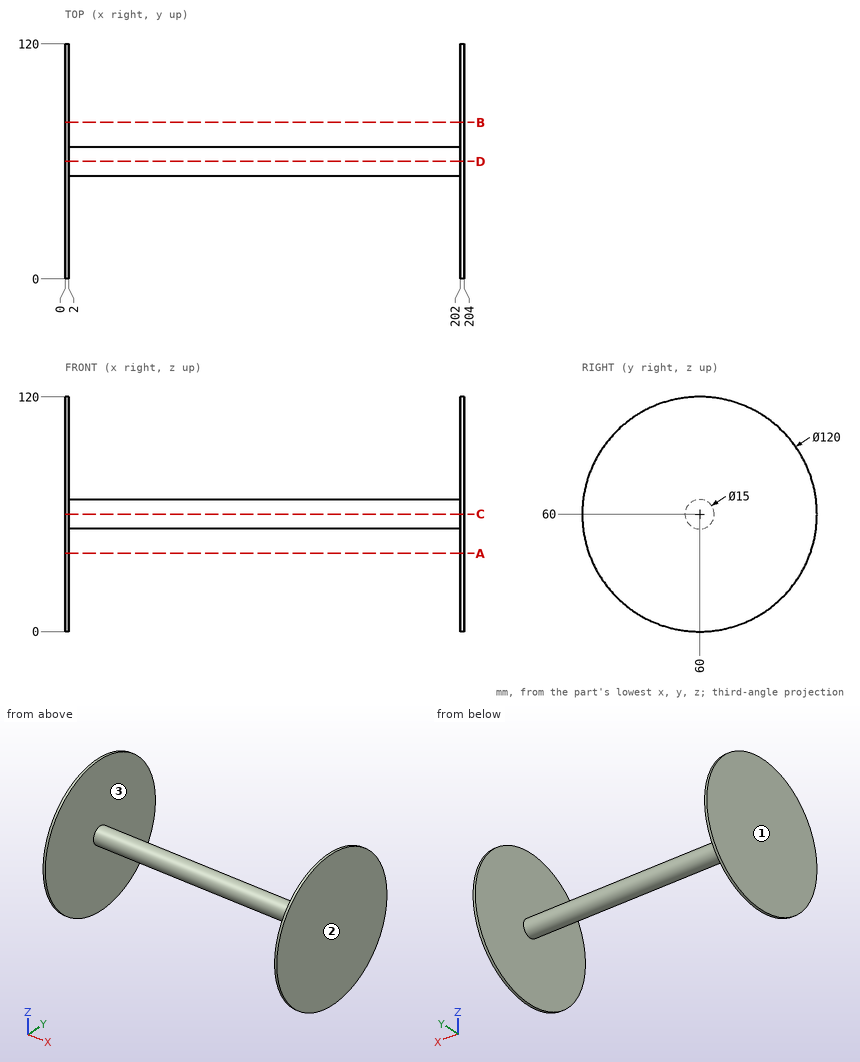
Design review of the part shown in the three views and the two pictorial views. Dimensions are in mm from the part's minimum x, y and z. Round coordinates to 2 decimals unless told otherwise and drop trailing zeros. Write each loop counter-clockwise with the first axis right and the second up, starting at its lowest first coordinate (ties: lowest second). Pieces come first, ordered by that corner, then holes. Notation, with made-up numbers: M -16,25 L 39,25 A19 cw 39,54 Z; hole C 53,5 d9. An arc over 180 degrees is marked long. Use a Markdown table: item, result. Add a question column.
Q1. To check wall thickness, follow line 1 (X direction, y = 92, z = 85). State the ranges of the line that lie inside material, in increasing order.
Q2. We need section C-C, the plane z = 60. State the section outline as (x, y) points, plus the area to 3 significant figures.
Q3. The part is to be moulded in two halves that separate along X. For the marked faces 1, 2 and 3, say which applies: pulls with the +X half, pulls with the -X half, needs draft (parallel to the pull), parting line crosses it, or undercut.
Q4. We need section A-A, the plane z = 40. State the section outline as (x, y) points, plus the area to 3 significant figures.
Q5. Insertion check: pin 1 (10 mm diameter, centred on x = 25.5, y = 69, fed in from -Z); pin 2 (1.5 mm diameter, centred on x = 117, y = 56.5, fed in from -Z); pin 3 (10 mm diameter, centred on y = 45, z = 101, fed in from -X); pin 4 (2 mm diameter, centred on x = 145.5, z = 57.5, fed in from -Y). Each pin has a flat end and moves straight along its axis. Give the tip position at first contact, or say it passes through.
Findings below:
| question | item | result |
|---|---|---|
| 1 | line 1 | x = 0 to 2, 202 to 204 |
| 2 | outline | M 0,0 L 2,0 L 2,52.5 L 202,52.5 L 202,0 L 204,0 L 204,120 L 202,120 L 202,67.5 L 2,67.5 L 2,120 L 0,120 Z |
| 2 | area | 3,480 mm² |
| 3 | face 1 | pulls with the -X half |
| 3 | face 2 | pulls with the +X half |
| 3 | face 3 | undercut |
| 4 | outline | M 0,3.43 L 2,3.43 L 2,116.57 L 0,116.57 Z; M 202,3.43 L 204,3.43 L 204,116.57 L 202,116.57 Z |
| 4 | area | 453 mm² |
| 5 | pin 1 | stops at z = 53.66 |
| 5 | pin 2 | stops at z = 53.02 |
| 5 | pin 3 | stops at x = 0 |
| 5 | pin 4 | stops at y = 52.65 |
